Here's how the part is built. I have some questions about the finished solid (model axes, mm). A direction names the side the tool comes from. Round coordinates to 2 decimals unless told otherwise and drop trailing zeros. Answer as a JSON object with one key per item and string values. Group by question number.
1) I want a section at A-A, the plane x = -42. Give the number of separate pieces and of enclosed holes in the cut face, then the cut area to 3 significant figures.
2) If I drill on line 1 along Z through (x, y) = (0.75, -370); line 2 along Z through (x, y) = (6, -370); line 3 along Y through (x, z) = (24, -16.5), over which ranges is the centre line in solid material (lowest first)? Write a range as [from, to].
3) If we mould it in two halves opening along Z, with no side actions, what happens to faces 5 (the face through (-1, -550.5, -23)), 6 (the face through (0, 0, 0)), 7 (the face through (-1.5, -439.2, 11.4))? For each: pulls with the +Z half, pulls with the -Z half, needs draft (parallel to the pull), parting line crosses it, or undercut.
4) Which directions (+Z, -Z, +X, -X, +Y, -Y) give clear straight access to the entire face, cutting with the end or side of a thin tool? Please do faces 1 (the face through (-19, -370, -18)), 2 (the face through (-13.887, -524.896, -10.648)), 3 (the face through (-0.78, -553.99, 32.47)), 4 (the face through (19, -370, -17)).
5) Will these pins go through, and if not, where does the flat tip stop? P1, Ø4, axis at x = 77.5, z = -61.5, coming from the -Y side; P2, Ø6, axis at x = -2, z = 29, coming from the -Y side; P3, Ø1.5, axis at x = -71, y = -552.5, coming from the -Z side.
from build123d import *

# Parameters (mm, degrees)
F0_R             = 11.5
F1_DEPTH         = 500
F2_R             = 17.5
F3_DEPTH         = 52
F5_R             = 17.5
F8_DEPTH         = 1.5
F10_R            = 11.5
F11_DEPTH        = 20
F12_R            = 3
F13_DEPTH        = 25
F14_R            = 6
F15_DEPTH        = 1
F15_COPIES_COUNT = 4
F16_R            = 4
F17_DEPTH        = 6
F17_COPIES_COUNT = 4
F19_DEPTH        = 4
F19_COPIES_COUNT = 4
F20_SIZE         = 0.5


# Not quite as in the source:
# - a pattern or mirror of a feature is missing from the dataset's text; its kind, count and spacing are read off the source's solid


with BuildPart() as f1:
    # F0 (on Front) → F1 (new body)
    with BuildSketch(Plane.XZ):
        Circle(F0_R)
    extrude(amount=F1_DEPTH)

    # F2 (on face) → F3 (join)
    with BuildSketch(Plane.XZ.offset(500)):
        Circle(F2_R)
    extrude(amount=F3_DEPTH)



with BuildPart() as f6:
    # F5 (on Right) → F6 (revolve)
    with BuildSketch(Plane.YZ):
        with Locations((-552, 110)):
            Circle(F5_R)
    revolve(axis=Axis((0, -586.2022111416, 0), (0, -1, 0)))


with BuildPart() as f1_1:
    add(f1.part)

    add(f6.part)  # F8 merges F6
    # F7 (on face) → F8 (join, symmetric)
    with BuildSketch(Plane.XZ.offset(552)):
        with BuildLine():
            ThreePointArc((-52.3712707503, -18.5), (-43.3414057713, -20.6545092961), (-36.2570335964, -26.6538461538))
            ThreePointArc((-36.2570335964, -26.6538461538), (-31.8198051534, -31.8198051534), (-26.6538461538, -36.2570335964))
            ThreePointArc((-26.6538461538, -36.2570335964), (-20.6545092961, -43.3414057713), (-18.5, -52.3712707503))
            Line((-18.5, -52.3712707503), (-18.5, -101.6479799574))
            ThreePointArc((-18.5, -101.6479799574), (0, -103.317771121), (18.5, -101.6479799574))
            Line((18.5, -101.6479799574), (18.5, -52.3712707503))
            ThreePointArc((18.5, -52.3712707503), (20.6545092961, -43.3414057713), (26.6538461538, -36.2570335964))
            ThreePointArc((26.6538461538, -36.2570335964), (31.8198051534, -31.8198051534), (36.2570335964, -26.6538461538))
            ThreePointArc((36.2570335964, -26.6538461538), (43.3414057713, -20.6545092961), (52.3712707503, -18.5))
            Line((52.3712707503, -18.5), (101.6479799574, -18.5))
            ThreePointArc((101.6479799574, -18.5), (103.317771121, 0), (101.6479799574, 18.5))
            Line((101.6479799574, 18.5), (52.3712707503, 18.5))
            ThreePointArc((52.3712707503, 18.5), (43.3414057713, 20.6545092961), (36.2570335964, 26.6538461538))
            ThreePointArc((36.2570335964, 26.6538461538), (0, 45), (-36.2570335964, 26.6538461538))
            ThreePointArc((-36.2570335964, 26.6538461538), (-43.3414057713, 20.6545092961), (-52.3712707503, 18.5))
            Line((-52.3712707503, 18.5), (-101.6479799574, 18.5))
            ThreePointArc((-101.6479799574, 18.5), (-103.317771121, 0), (-101.6479799574, -18.5))
            Line((-101.6479799574, -18.5), (-52.3712707503, -18.5))
        make_face()
    extrude(amount=F8_DEPTH, both=True)

    # F10 (on offset) → F11 (join)
    with BuildSketch(Plane(origin=(0, -380, 0), x_dir=(-1, 0, 0), z_dir=(0, 1, 0))):
        with BuildLine():
            Line((19, -35), (19, 0))
            ThreePointArc((19, 0), (0, 19), (-19, 0))
            Line((-19, 0), (-19, -35))
            Line((-19, -35), (19, -35))
        make_face()
        Circle(F10_R, mode=Mode.SUBTRACT)
    extrude(amount=F11_DEPTH)

    # F12 (on face) → F13 (cut)
    with BuildSketch(Plane.YZ.offset(19)):
        with Locations((-370, -28)):
            Circle(F12_R)
    extrude(amount=-F13_DEPTH, mode=Mode.SUBTRACT)

    # F14 (on face) → F15 (join)
    with BuildSketch(Plane.XZ.offset(553.5)):
        with Locations((0, 26.5213046223)):
            Circle(F14_R)
    f15 = extrude(amount=F15_DEPTH)

    # F15_copies: F15 ×4 about axis
    f15_copies_axis = Axis((0, 0, 0), (0, 1, 0))
    for i in range(1, F15_COPIES_COUNT):
        add(f15.rotate(f15_copies_axis, i * 360 / F15_COPIES_COUNT))

    # F16 (on face) → F17 (join)
    with BuildSketch(Plane.XZ.offset(554.5)):
        with Locations((0, 26.5213046223)):
            Circle(F16_R)
    f17 = extrude(amount=F17_DEPTH)

    # F17_copies: F17 ×4 about axis
    f17_copies_axis = Axis((0, 0, 0), (0, 1, 0))
    for i in range(1, F17_COPIES_COUNT):
        add(f17.rotate(f17_copies_axis, i * 360 / F17_COPIES_COUNT))

    # F18 (on face) → F19 (cut)
    with BuildSketch(Plane.XZ.offset(560.5)):
        Polygon((2.9804941814, 26.7480426348), (1.2938862119, 29.2158573055), (-1.6866079695, 28.989119293), (-2.9804941814, 26.2945666098), (-1.2938862119, 23.8267519391), (1.6866079695, 24.0534899516), align=None)
    f19 = extrude(amount=-F19_DEPTH, mode=Mode.SUBTRACT)

    # F19_copies: F19 ×4 about axis
    f19_copies_axis = Axis((0, 0, 0), (0, 1, 0))
    for i in range(1, F19_COPIES_COUNT):
        add(f19.rotate(f19_copies_axis, i * 360 / F19_COPIES_COUNT), mode=Mode.SUBTRACT)

    # F20
    f20_edges = [f1_1.edges().sort_by_distance(p)[0] for p in [
        (-4, -560.5, 26.521305),
        (-26.521305, -560.5, -4),
        (4, -560.5, -26.521305),
        (26.521305, -560.5, 4),
    ]]
    chamfer(f20_edges, length=F20_SIZE)


solid = f1_1.part
Outcome:
{
 "1": {"separate pieces": "3", "enclosed holes": "0", "area": "2,210 mm^2"},
 "2": {"line 1": "[-35, -31], [-25, 18.99]", "line 2": "[-35, -31], [-25, 18.03]", "line 3": "[-553.5, -550.5]"},
 "3": {"face 5": "undercut", "face 6": "needs draft", "face 7": "parting line crosses it"},
 "4": {"face 1": "+Z, -Z, -X, +Y", "face 2": "none", "face 3": "-Y", "face 4": "+Z, -Z, +X, +Y"},
 "5": {"P1": "y = -566.97", "P2": "y = -560.5", "P3": "z = -106.39"}
}
